For this review, take the finished solid that the model builds, in its own axes (mm). A direction names the side the tool comes from. Round coordinates to 2 decimals unless told otherwise and drop trailing zeros. Write each loop counter-clockwise with the first axis right and the second up, starting at its lowest first coordinate (ties: lowest second). Pieces come first, ordered by that corner, then holes. Notation, with made-up numbers: (81.5, 68) - (130.5, 68) arc R25 ccw to (130.5, 81) - close; hole circle Ø6 at (57.25, 40.25). An arc over 180 degrees is marked (long way). One line per item, written item: value. Start each with the question number.
Q1. Add section B-B on x = 0. Write out the cut boundary in (y, z).
Q2. Add section C-C on y = 13.5. Write out the cut boundary in (x, z), and give its area (3 significant figures).
Q3. For probe 1 along Z at (x, y) = (0, 18); probe 2 along Z at (x, y) = (0, 0.45); probe 3 along Y at (x, z) = (-4.5, 2.25), list the stretches that pass through material, from the lowest coordinate up.
Q4. Clearance check with flat-ended pins moving along their axes: pin 1 Ø5 at (x, z) = (0, 0) entering from -Y; pin 2 Ø1.4 at (x, z) = (0, 0) entering from +Y; pin 3 Ø1 at (x, y) = (2.5, 8.5) entering from +Z; pin 4 Ø1 at (y, z) = (16, 3) entering from +X. State where each tip first meets the part, or that it passes through.
Q5. Tool access review of faces 1 (the face through (0, 1.5, 0)), 2 (the face through (0, 0, -1)), 3 (the face through (3.905, 12.374, -0.867)): name each direction out of +Z, -Z, +X, -X, +Y, -Y from which nothing blocks a thin tool from reaching the whole face with its end or side.
Q6. Add section D-D on x = 2.25. Write out the cut boundary in (y, z).
Q7. Mouldability with a two-part tool opening along Z and no side actions: class faces 4 (the face through (-0.03, 0.76, 0.75)), 5 (the face through (-1.42, 21.5, -3.92)), 6 (the face through (-6, 12, 0)) as +Z half, -Z half, draft (parallel to the pull), parting line (faces both ways), or undercut.
Q8. Add section A-A on z = 0. Write out the cut boundary in (x, y), and give its area (3 significant figures).
Autodesk Inventor part; units mm, degrees
ref_plane "YZ Plane" through (0, 0, 0) normal (1, 0, 0) x (0, 1, 0)
ref_plane "XZ Plane" through (0, 0, 0) normal (0, 1, 0) x (-1, 0, 0)
ref_plane "XY Plane" through (0, 0, 0) normal (0, 0, 1) x (1, 0, 0)
sketch "Skizze2" plane through (0, 0, 0) normal (0, 0, 1) x (1, 0, 0)
  line L0 (0, 0) -> (4.5, 0)
  line L1 (4.5, 0) -> (4.5, 1.5)
  line L2 (4.5, 1.5) -> (6, 1.5)
  line L3 (6, 1.5) -> (6, 21.5)
  line L4 (6, 21.5) -> (0, 21.5)
  line L5 (0, 21.5) -> (0, 0)
  point P0 (2.25, 0)
  point P1 (5.25, 1.5)
  dimension "d1" = 21.5
  dimension "d2" = 1.5
  dimension "d3" = 12
  dimension "d4" = 9
revolve "Umdrehung1" add sketch "Skizze2" angle 360 about axis through (0, 21.5, 0) along (0, -1, 0)
sketch "Skizze3" plane through (0, 21.5, 0) normal (0, 1, 0) x (1, 0, 0)
  circle A0 centre (0, 0) radius 6
hole "Bohrung1" at (0, 21.5, 0) direction (0, -1, 0) diameter 8 depth 18
sketch "Sketch4" plane through (0, 0, 0) normal (0, -1, 0) x (1, 0, 0)
  circle A0 centre (0, 0) radius 4.5
hole "Hole2" at (0, 0, 0) direction (0, 1, 0) diameter 1.5 depth 1.5
properties part number "153 part 1" material "Gold"
Result set:
1. outline: (0, -4.5) - (1.5, -4.5) - (1.5, -6) - (21.5, -6) - (21.5, -4) - (3.5, -4) - (3.5, 4) - (21.5, 4) - (21.5, 6) - (1.5, 6) - (1.5, 4.5) - (0, 4.5) - (0, 0.75) - (1.5, 0.75) - (1.5, -0.75) - (0, -0.75) - close
2. outline: circle Ø12 at (0, 0); hole circle Ø8 at (0, 0)
2. area: 62.8 mm^2
3. probe 1: z = -6 to -4, 4 to 6
3. probe 2: z = -4.5 to -0.75, 0.75 to 4.5
3. probe 3: y = 1.5 to 21.5
4. pin 1: stops at y = 0
4. pin 2: stops at y = 3.5
4. pin 3: stops at z = 5.66
4. pin 4: stops at x = 5.45
5. face 1: -Y
5. face 2: +Z, -Z, +X, -X, -Y
5. face 3: +Y
6. outline: (0, -3.9) - (1.5, -3.9) - (1.5, -5.56) - (21.5, -5.56) - (21.5, -3.31) - (3.5, -3.31) - (3.5, 3.31) - (21.5, 3.31) - (21.5, 5.56) - (1.5, 5.56) - (1.5, 3.9) - (0, 3.9) - close
7. face 4: undercut
7. face 5: draft
7. face 6: parting line
8. outline: (-6, 1.5) - (-4.5, 1.5) - (-4.5, 0) - (-0.75, 0) - (-0.75, 1.5) - (0.75, 1.5) - (0.75, 0) - (4.5, 0) - (4.5, 1.5) - (6, 1.5) - (6, 21.5) - (4, 21.5) - (4, 3.5) - (-4, 3.5) - (-4, 21.5) - (-6, 21.5) - close
8. area: 107 mm^2
